Input: part model. Units: mm. Frame: model coordinates. A direction names the side the tool comes from. Coordinates: 2 decimals unless noted, no trailing zeros. Loops run counter-clockwise (first coordinate to the right, second up) from the corner with the lowest first, then second, coordinate; pieces in that order, holes last.
Item 1: Section B-B on x = 76. Return loops of the section in (y, z), and give its area (3 significant figures).
Item 2: Section A-A on x = -76. Return loops of the section in (y, z), and give its area (3 significant figures).
Item 3: Contact query for flat-ended pins moving along their axis: P1, Ø3, axis at x = -60, z = -5.5, coming from the +Y side; P2, Ø11, axis at x = -75.5, z = -12.5, coming from the +Y side; P3, Ø3, axis at x = 28, z = -11.5, coming from the +Y side. Output: stop coordinate, or through.
Item 4: Pull-direction query (X, two-part tool) for faces 3 (the flat face through (29, -34.965, 0)), 4 (the cylindrical face through (-99.67, -38.88, -0.35)), 5 (the flat face through (-12, -24, -25)); classes: released by +X, released by -X, zero draft, split by the parting line, or undercut.
Item 5: Ray query, line 1 along Y through (x, z) = (47.5, -2); line 2 along Y through (x, z) = (-37, -12.5); line 3 along Y through (x, z) = (-83, 2). Return the intervals inside material, ascending.
Item 6: Reachability of faces 1 (the flat face through (15.627, -12.78, 0.35)), 2 (the flat face through (6, 10.035, 0)) from +Z, -Z, +X, -X, +Y, -Y: full face, straight path, thin tool, end or side. Return the list, or none.
Item 7: Section C-C on y = -26.5. Give the number of separate pieces and of enclosed holes in the cut face, and give its area (3 significant figures).
```python
from build123d import *

# Parameters (mm, degrees)
F1_DEPTH     = 25
F2_T1_DEPTH  = 30
F2_T3_DEPTH  = 30
F2_T5_DEPTH  = 30
F2_T7_DEPTH  = 30
F2_T9_DEPTH  = 30
F2_T11_DEPTH = 30
F2_T13_DEPTH = 30
F2_T15_DEPTH = 30
F2_T17_DEPTH = 30
F2_T19_DEPTH = 30
F2_T21_DEPTH = 30
F2_T23_DEPTH = 60.3553390593
F2_T25_DEPTH = 75


# Not quite as in the source:
# - a fillet or chamfer that OpenCascade refuses, or shapes differently, is made with other operations: its cross-section is extruded or revolved along the edge and cut away or added


with BuildPart() as f1:
    # F0 (on Top) → F1 (new body, symmetric)
    with BuildSketch(Plane.XY):
        Polygon((-56.5580020845, 10.0351088219), (-69.7381969311, -3.1450860247), (-101.5580020845, -34.9648911781), (-96.5580020845, -34.9648911781), (-51.5580020845, 10.0351088219), align=None)
        Polygon((-96.5580020845, -34.9648911781), (-101.5580020845, -34.9648911781), (-101.5580020845, -39.9648911781), (53.4419979155, -39.9648911781), (53.4419979155, -34.9648911781), (48.4419979155, -34.9648911781), (38.4419979155, -34.9648911781), (33.4419979155, -34.9648911781), (23.4419979155, -34.9648911781), (18.4419979155, -34.9648911781), (8.4419979155, -34.9648911781), (3.4419979155, -34.9648911781), (-6.5580020845, -34.9648911781), (-11.5580020845, -34.9648911781), (-21.5580020845, -34.9648911781), (-26.5580020845, -34.9648911781), (-36.5580020845, -34.9648911781), (-41.5580020845, -34.9648911781), (-51.5580020845, -34.9648911781), (-56.5580020845, -34.9648911781), (-66.5580020845, -34.9648911781), (-71.5580020845, -34.9648911781), (-81.5580020845, -34.9648911781), (-86.5580020845, -34.9648911781), align=None)
        Polygon((-41.5580020845, 10.0351088219), (-86.5580020845, -34.9648911781), (-81.5580020845, -34.9648911781), (-36.5580020845, 10.0351088219), align=None)
        Polygon((48.4419979155, -34.9648911781), (53.4419979155, -34.9648911781), (98.4419979155, 10.0351088219), (93.4419979155, 10.0351088219), align=None)
        Polygon((-26.5580020845, 10.0351088219), (-71.5580020845, -34.9648911781), (-66.5580020845, -34.9648911781), (-21.5580020845, 10.0351088219), align=None)
        Polygon((33.4419979155, -34.9648911781), (38.4419979155, -34.9648911781), (83.4419979155, 10.0351088219), (78.4419979155, 10.0351088219), align=None)
        Polygon((-11.5580020845, 10.0351088219), (-56.5580020845, -34.9648911781), (-51.5580020845, -34.9648911781), (-6.5580020845, 10.0351088219), align=None)
        Polygon((18.4419979155, -34.9648911781), (23.4419979155, -34.9648911781), (68.4419979155, 10.0351088219), (63.4419979155, 10.0351088219), align=None)
        Polygon((3.4419979155, 10.0351088219), (-41.5580020845, -34.9648911781), (-36.5580020845, -34.9648911781), (8.4419979155, 10.0351088219), align=None)
        Polygon((3.4419979155, -34.9648911781), (8.4419979155, -34.9648911781), (53.4419979155, 10.0351088219), (48.4419979155, 10.0351088219), align=None)
        Polygon((18.4419979155, 10.0351088219), (-26.5580020845, -34.9648911781), (-21.5580020845, -34.9648911781), (23.4419979155, 10.0351088219), align=None)
        Polygon((-11.5580020845, -34.9648911781), (-6.5580020845, -34.9648911781), (38.4419979155, 10.0351088219), (33.4419979155, 10.0351088219), align=None)
    extrude(amount=F1_DEPTH, both=True)

    # F2: fillet of radius 5 on 25 edges, made by hand

    # F2_s2 → F2_t1 (cut)
    with BuildSketch(Plane.YZ.offset(-69.0580020845)):
        with BuildLine():
            ThreePointArc((10.0351088219, -20), (8.5706427278, -23.5355339059), (5.0351088219, -25))
            Line((5.0351088219, -25), (10.0351088219, -25))
            Line((10.0351088219, -25), (10.0351088219, -20))
        make_face()
        with BuildLine():
            ThreePointArc((10.0351088219, 20), (8.5706427278, 23.5355339059), (5.0351088219, 25))
            Line((5.0351088219, 25), (10.0351088219, 25))
            Line((10.0351088219, 25), (10.0351088219, 20))
        make_face()
    extrude(amount=F2_T1_DEPTH, mode=Mode.SUBTRACT)

    # F2_s4 → F2_t3 (cut)
    with BuildSketch(Plane.YZ.offset(-54.0580020845)):
        with BuildLine():
            ThreePointArc((10.0351088219, 20), (8.5706427278, 23.5355339059), (5.0351088219, 25))
            Line((5.0351088219, 25), (10.0351088219, 25))
            Line((10.0351088219, 25), (10.0351088219, 20))
        make_face()
        with BuildLine():
            ThreePointArc((10.0351088219, -20), (8.5706427278, -23.5355339059), (5.0351088219, -25))
            Line((5.0351088219, -25), (10.0351088219, -25))
            Line((10.0351088219, -25), (10.0351088219, -20))
        make_face()
    extrude(amount=F2_T3_DEPTH, mode=Mode.SUBTRACT)

    # F2_s6 → F2_t5 (cut)
    with BuildSketch(Plane.YZ.offset(-39.0580020845)):
        with BuildLine():
            ThreePointArc((10.0351088219, -20), (8.5706427278, -23.5355339059), (5.0351088219, -25))
            Line((5.0351088219, -25), (10.0351088219, -25))
            Line((10.0351088219, -25), (10.0351088219, -20))
        make_face()
        with BuildLine():
            ThreePointArc((10.0351088219, 20), (8.5706427278, 23.5355339059), (5.0351088219, 25))
            Line((5.0351088219, 25), (10.0351088219, 25))
            Line((10.0351088219, 25), (10.0351088219, 20))
        make_face()
    extrude(amount=F2_T5_DEPTH, mode=Mode.SUBTRACT)

    # F2_s8 → F2_t7 (cut)
    with BuildSketch(Plane.YZ.offset(-24.0580020845)):
        with BuildLine():
            ThreePointArc((10.0351088219, 20), (8.5706427278, 23.5355339059), (5.0351088219, 25))
            Line((5.0351088219, 25), (10.0351088219, 25))
            Line((10.0351088219, 25), (10.0351088219, 20))
        make_face()
        with BuildLine():
            ThreePointArc((10.0351088219, -20), (8.5706427278, -23.5355339059), (5.0351088219, -25))
            Line((5.0351088219, -25), (10.0351088219, -25))
            Line((10.0351088219, -25), (10.0351088219, -20))
        make_face()
    extrude(amount=F2_T7_DEPTH, mode=Mode.SUBTRACT)

    # F2_s10 → F2_t9 (cut)
    with BuildSketch(Plane.YZ.offset(-9.0580020845)):
        with BuildLine():
            ThreePointArc((10.0351088219, 20), (8.5706427278, 23.5355339059), (5.0351088219, 25))
            Line((5.0351088219, 25), (10.0351088219, 25))
            Line((10.0351088219, 25), (10.0351088219, 20))
        make_face()
        with BuildLine():
            ThreePointArc((10.0351088219, -20), (8.5706427278, -23.5355339059), (5.0351088219, -25))
            Line((5.0351088219, -25), (10.0351088219, -25))
            Line((10.0351088219, -25), (10.0351088219, -20))
        make_face()
    extrude(amount=F2_T9_DEPTH, mode=Mode.SUBTRACT)

    # F2_s12 → F2_t11 (cut)
    with BuildSketch(Plane.YZ.offset(5.9419979155)):
        with BuildLine():
            ThreePointArc((10.0351088219, -20), (8.5706427278, -23.5355339059), (5.0351088219, -25))
            Line((5.0351088219, -25), (10.0351088219, -25))
            Line((10.0351088219, -25), (10.0351088219, -20))
        make_face()
        with BuildLine():
            ThreePointArc((10.0351088219, 20), (8.5706427278, 23.5355339059), (5.0351088219, 25))
            Line((5.0351088219, 25), (10.0351088219, 25))
            Line((10.0351088219, 25), (10.0351088219, 20))
        make_face()
    extrude(amount=F2_T11_DEPTH, mode=Mode.SUBTRACT)

    # F2_s14 → F2_t13 (cut)
    with BuildSketch(Plane.YZ.offset(20.9419979155)):
        with BuildLine():
            ThreePointArc((10.0351088219, 20), (8.5706427278, 23.5355339059), (5.0351088219, 25))
            Line((5.0351088219, 25), (10.0351088219, 25))
            Line((10.0351088219, 25), (10.0351088219, 20))
        make_face()
        with BuildLine():
            ThreePointArc((10.0351088219, -20), (8.5706427278, -23.5355339059), (5.0351088219, -25))
            Line((5.0351088219, -25), (10.0351088219, -25))
            Line((10.0351088219, -25), (10.0351088219, -20))
        make_face()
    extrude(amount=F2_T13_DEPTH, mode=Mode.SUBTRACT)

    # F2_s16 → F2_t15 (cut)
    with BuildSketch(Plane.YZ.offset(35.9419979155)):
        with BuildLine():
            ThreePointArc((10.0351088219, 20), (8.5706427278, 23.5355339059), (5.0351088219, 25))
            Line((5.0351088219, 25), (10.0351088219, 25))
            Line((10.0351088219, 25), (10.0351088219, 20))
        make_face()
        with BuildLine():
            ThreePointArc((10.0351088219, -20), (8.5706427278, -23.5355339059), (5.0351088219, -25))
            Line((5.0351088219, -25), (10.0351088219, -25))
            Line((10.0351088219, -25), (10.0351088219, -20))
        make_face()
    extrude(amount=F2_T15_DEPTH, mode=Mode.SUBTRACT)

    # F2_s18 → F2_t17 (cut)
    with BuildSketch(Plane.YZ.offset(50.9419979155)):
        with BuildLine():
            ThreePointArc((10.0351088219, 20), (8.5706427278, 23.5355339059), (5.0351088219, 25))
            Line((5.0351088219, 25), (10.0351088219, 25))
            Line((10.0351088219, 25), (10.0351088219, 20))
        make_face()
        with BuildLine():
            ThreePointArc((10.0351088219, -20), (8.5706427278, -23.5355339059), (5.0351088219, -25))
            Line((5.0351088219, -25), (10.0351088219, -25))
            Line((10.0351088219, -25), (10.0351088219, -20))
        make_face()
    extrude(amount=F2_T17_DEPTH, mode=Mode.SUBTRACT)

    # F2_s20 → F2_t19 (cut)
    with BuildSketch(Plane.YZ.offset(65.9419979155)):
        with BuildLine():
            ThreePointArc((10.0351088219, 20), (8.5706427278, 23.5355339059), (5.0351088219, 25))
            Line((5.0351088219, 25), (10.0351088219, 25))
            Line((10.0351088219, 25), (10.0351088219, 20))
        make_face()
        with BuildLine():
            ThreePointArc((10.0351088219, -20), (8.5706427278, -23.5355339059), (5.0351088219, -25))
            Line((5.0351088219, -25), (10.0351088219, -25))
            Line((10.0351088219, -25), (10.0351088219, -20))
        make_face()
    extrude(amount=F2_T19_DEPTH, mode=Mode.SUBTRACT)

    # F2_s22 → F2_t21 (cut)
    with BuildSketch(Plane.YZ.offset(80.9419979155)):
        with BuildLine():
            ThreePointArc((10.0351088219, 20), (8.5706427278, 23.5355339059), (5.0351088219, 25))
            Line((5.0351088219, 25), (10.0351088219, 25))
            Line((10.0351088219, 25), (10.0351088219, 20))
        make_face()
        with BuildLine():
            ThreePointArc((10.0351088219, -20), (8.5706427278, -23.5355339059), (5.0351088219, -25))
            Line((5.0351088219, -25), (10.0351088219, -25))
            Line((10.0351088219, -25), (10.0351088219, -20))
        make_face()
    extrude(amount=F2_T21_DEPTH, mode=Mode.SUBTRACT)

    # F2_s24 → F2_t23 (cut)
    with BuildSketch(Plane.XY.offset(-30.1776695297)):
        with BuildLine():
            ThreePointArc((-100.0935359904, -33.5004250841), (-101.1773997471, -35.1225418282), (-101.5580020845, -37.03595899))
            Line((-101.5580020845, -37.03595899), (-101.5580020845, -34.9648911781))
            Line((-101.5580020845, -34.9648911781), (-100.0935359904, -33.5004250841))
        make_face()
    extrude(amount=F2_T23_DEPTH, mode=Mode.SUBTRACT)

    # F2_s26 → F2_t25 (cut)
    with BuildSketch(Plane.XY.offset(-37.5)):
        with BuildLine():
            ThreePointArc((-96.5580020845, -39.9648911781), (-100.0935359904, -38.5004250841), (-101.5580020845, -34.9648911781))
            Line((-101.5580020845, -34.9648911781), (-101.5580020845, -39.9648911781))
            Line((-101.5580020845, -39.9648911781), (-96.5580020845, -39.9648911781))
        make_face()
        with BuildLine():
            ThreePointArc((53.4419979155, -34.9648911781), (51.9775318214, -38.5004250841), (48.4419979155, -39.9648911781))
            Line((48.4419979155, -39.9648911781), (53.4419979155, -39.9648911781))
            Line((53.4419979155, -39.9648911781), (53.4419979155, -34.9648911781))
        make_face()
    extrude(amount=F2_T25_DEPTH, mode=Mode.SUBTRACT)


solid = f1.part
```
Results found:
1. outline: (-12.41, -25) - (-7.41, -25) - (-7.41, 25) - (-12.41, 25) - close; (2.59, -25) - (5.04, -25) arc R5 ccw to (7.59, -24.3) - (7.59, 24.3) arc R5 ccw to (5.04, 25) - (2.59, 25) - close
1. area: 499 mm2
2. outline: (-39.96, -25) - (-34.96, -25) - (-34.96, 25) - (-39.96, 25) - close; (-29.41, -25) - (-24.41, -25) - (-24.41, 25) - (-29.41, 25) - close; (-14.41, -25) - (-9.41, -25) - (-9.41, 25) - (-14.41, 25) - close
2. area: 750 mm2
3. P1: stops at y = 8.09
3. P2: stops at y = -3.41
3. P3: stops at y = 6.09
4. face 3: undercut
4. face 4: released by -X
4. face 5: zero draft
5. line 1: y = -39.96 to -34.96, -25.91 to -20.91, -10.91 to -5.91, 4.09 to 9.09
5. line 2: y = -39.96 to -30.41, -20.41 to -15.41, -5.41 to -0.41, 9.59 to 10.04
5. line 3: y = -39.96 to -31.41, -21.41 to -16.41
6. face 1: +Z, -Z
6. face 2: +Z, -Z, +X, -X, +Y
7. separate pieces: 11
7. enclosed holes: 0
7. area: 2,750 mm2
